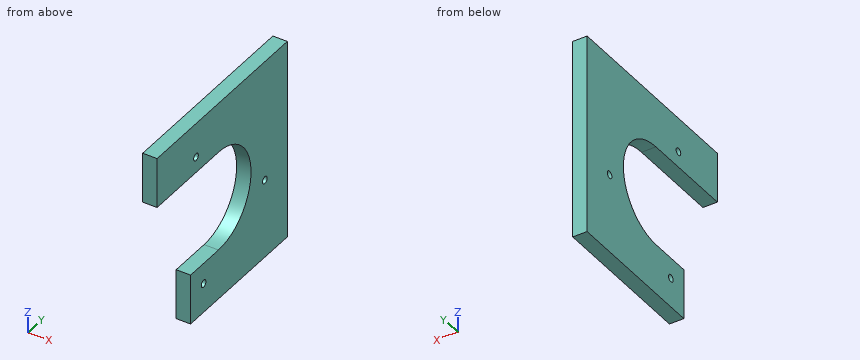
Autodesk Inventor part; units mm, degrees
ref_plane "РабПлоскость8" through (-15, 0, 0) normal (-1, 0, 0) x (0, 0, 1)
ref_plane "РабПлоскость7" through (-25, 0, 0) normal (-1, 0, 0) x (0, 0, 1)
ref_plane "YZ Plane" through (0, 0, 0) normal (1, 0, 0) x (0, 1, 0)
ref_plane "РабПлоскость8" through (-15, 0, 0) normal (-1, 0, 0) x (0, 0, 1)
sketch "Эскиз6" plane through (-15, 0, 0) normal (-1, 0, 0) x (0, 0, 1)
  line L0 (0, 0) -> (0, -66)
  line L1 (0, -66) -> (-70, -66)
  line L2 (-70, -66) -> (-70, 74)
  line L3 (-70, 74) -> (70, 74)
  line L4 (70, 74) -> (70, -66)
  line L5 (70, -66) -> (0, -66)
  circle A0 centre (0, 0) radius 3
  circle A1 centre (-14.8513, 49.8341) radius 2.5
  circle A2 centre (0, 0) radius 52
  line L6 (70, 0) -> (70, 30)
  line L7 (70, 0) -> (70, -20)
  circle A3 centre (0, 0) radius 35
  circle A4 centre (0, 0) radius 35
  line L8 (0, 0) -> (70, 0)
  circle A5 centre (-14.8513, 49.8341) radius 2.5
  line L9 (-70, 74) -> (-73, 74)
  line L10 (-70, 89) -> (-70, 74)
  line L11 (-70, 74) -> (-67, 74)
  line L12 (-67, 74) -> (-67, 89)
  line L13 (-67, 89) -> (-70, 89)
  line L14 (-70, -66) -> (-70, -81)
  line L15 (-70, -81) -> (-67, -81)
  line L16 (-67, -81) -> (-67, -66)
  circle A6 centre (46.0282, -24.1951) radius 2.5
  circle A7 centre (46.0282, -24.1951) radius 2.5
  line L17 (0, 74) -> (-30, 74)
  line L18 (-35, 0) -> (-35, 74)
  line L19 (-35, 0) -> (-35, -30)
  line L20 (-35, -30) -> (-70, -30)
  line L21 (35, 0) -> (35, -66)
  arc A8 (-56.6592, -9.0725) -> (-41.4997, -22.0629) centre (-49.4698, -16.0232) ccw
  circle A9 centre (-49.4698, -16.0232) radius 2.5
  point P0 (-1.4375, -51.9801)
  point P1 (38.1911, 35.2908)
  point P2 (0, -35)
  point P3 (35, 0)
  dimension "d36" = 66
  dimension "d37" = 70
  dimension "d38" = 140
  dimension "d39" = 140
  dimension "d45" = 3
  dimension "d46" = 15
  dimension "d47" = 15
  dimension "d48" = 3
  dimension "d49" = 30
  dimension "d54" = 30
extrude "Выдавливание5" add sketch "Эскиз6" along normal blind 10 contours A3 L18 A2 A1 L8 | L8 A2 A6 L21 | L19 L20 A2 A9 L18 | L8 L4 L5 L21 A2 A6 | A2 A1 L18 L3 L4 L8 | L20 L2 L3 L18 A2 A9
ref_plane "РабПлоскость7" through (-25, 0, 0) normal (-1, 0, 0) x (0, 0, 1)
sketch "Эскиз7" plane through (-25, 0, 0) normal (-1, 0, 0) x (0, 0, 1)
  line L0 (-70, 74) -> (-70, -30)
  line L1 (-70, -30) -> (-35, -30)
  line L2 (-35, -30) -> (-35, 0)
  circle A0 centre (-49.4698, -16.0232) radius 2.5
  arc A1 (35, 0) -> (-35, 0) centre (0, 0) ccw
  line L3 (70, 74) -> (-70, 74)
  line L4 (70, -66) -> (70, 74)
  line L5 (35, 0) -> (35, -66)
  line L6 (35, -66) -> (70, -66)
  circle A2 centre (46.0282, -24.1951) radius 2.5
  circle A3 centre (-14.8513, 49.8341) radius 2.5
  circle A4 centre (0, 0) radius 3
  circle A5 centre (-14.8513, 49.8341) radius 2.5
  circle A6 centre (0, 0) radius 52
  circle A7 centre (0, 0) radius 43.5
  circle A8 centre (0, 0) radius 43.5
  circle A9 centre (46.0282, -24.1951) radius 2.5
  line L7 (0, 0) -> (46.0282, -24.1951)
  line L8 (46.0282, -24.1951) -> (46.0282, 0)
  line L9 (-14.8513, 49.8341) -> (0, 49.8341)
  arc A10 (28.4229, 37.4318) -> (-5.3572, 46.6937) centre (0, 0) ccw
  line L10 (0, 49.8341) -> (0, 0)
  circle A11 centre (-49.4698, -16.0232) radius 2.5
  line L11 (0, 0) -> (-49.4698, -16.0232)
  line L12 (-49.4698, -16.0232) -> (-49.4995, -0.2197)
  circle A12 centre (-51.9995, -0.2244) radius 2.5
  dimension "d57" = 104
  dimension "d55" = 104
  dimension "d56" = 140
  dimension "d58" = 35
  dimension "d59" = 87
  dimension "d60" = 24.1951
  dimension "d61" = 46.0282
  dimension "d62" = 49.8341
  dimension "d63" = 14.8513
  dimension "d64" = 15.8034
  dimension "d65" = 49.4999
properties part number "Двигатель ущербный"
Input: part model. Units: mm. Frame: model coordinates. Coordinates: 2 decimals unless noted, no trailing zeros. Loops run counter-clockwise (first coordinate to the right, second up) from the corner with the lowest first, then second, coordinate; pieces in that order, holes last.
(1) Section B-B on x = -17. Return the cut outline in (y, z).
(2) Material intervals for probe 1 along Z at (x, y) = (-16.25, -28); probe 2 along Y at (x, z) = (-23.5, -45); probe 3 along Z at (x, y) = (-22.25, -54), sorted ascending.
(3) First-contact query: pin 1 Ø3 at (y, z) = (-16.02, -49.47) entering from +X. Flat tip, straight axial feed; report the tip coordinate or a pass-through.
(4) Section C-C on z = 0. Return the cut outline in (x, y).
(5) Section D-D on y = 27. Return the cut outline in (x, z).
(6) Section A-A on y = -9. Return the cut outline in (x, z).
Data:
1. outline: (-66, 35) - (0, 35) arc R35 cw to (0, -35) - (-30, -35) - (-30, -70) - (74, -70) - (74, 70) - (-66, 70) - close; hole circle Ø5 at (-24.2, 46.03); hole circle Ø5 at (-16.02, -49.47); hole circle Ø5 at (49.83, -14.85)
2. probe 1: z = -70 to -35, 35 to 70
2. probe 2: y = -30 to 74
2. probe 3: z = 35 to 70
3. pin 1: passes through
4. outline: (-25, 35) - (-15, 35) - (-15, 74) - (-25, 74) - close
5. outline: (-25, -70) - (-15, -70) - (-15, -22.27) - (-25, -22.27) - close; (-25, 22.27) - (-15, 22.27) - (-15, 70) - (-25, 70) - close
6. outline: (-25, -70) - (-15, -70) - (-15, -35) - (-25, -35) - close; (-25, 35) - (-15, 35) - (-15, 70) - (-25, 70) - close
